Design review of the part built by this model. Coordinates are the model's own, in mm. A direction names the side the tool comes from. Round coordinates to 2 decimals unless told otherwise and drop trailing zeros. Order: outer loops, then holes, each group sorted by start corner. A loop starts at its lowest first (then second) coordinate and runs counter-clockwise, first axis right, second up.
from build123d import *

# Parameters (mm, degrees)
SKETCH1_R           = 2.2
BOSS_EXTRUDE1_DEPTH = 2.38125
BOSS_EXTRUDE3_DEPTH = 2.38125
SKETCH4_R           = 2.15265
CUT_EXTRUDE1_DEPTH  = 2.38125
FILLET2_R           = 2.38125


with BuildPart() as part:
    # Sketch1 → Boss-Extrude1 (new body)
    # profile 1 of 2: a face of its own
    with BuildSketch(Plane(origin=(0, 0, 0), x_dir=(1, 0, 0), z_dir=(0, 1, 0))):
        Polygon((0, -6.985), (0, 0), (-20.15, 0), (-20.15, 20), (-27.65, 20), (-27.65, -6.985), align=None)
        with Locations(Location((-23.9, 4.9, 0), (0, 0, 90))):
            Circle(SKETCH1_R, mode=Mode.SUBTRACT)
        with Locations(Location((-23.9, 15.1, 0), (0, 0, 90))):
            Circle(SKETCH1_R, mode=Mode.SUBTRACT)
    # profile 2 of 2: a face of its own
    with BuildSketch(Plane(origin=(0, 0, 0), x_dir=(1, 0, 0), z_dir=(0, 1, 0))):
        Polygon((20.15, 20), (20.15, 0), (0, 0), (0, -6.985), (27.65, -6.985), (42.38375, -6.985), (42.38375, 20), align=None)
        with Locations(Location((23.9, 4.9, 0), (0, 0, 90))):
            Circle(SKETCH1_R, mode=Mode.SUBTRACT)
        with Locations(Location((23.9, 15.1, 0), (0, 0, 90))):
            Circle(SKETCH1_R, mode=Mode.SUBTRACT)
    extrude(amount=BOSS_EXTRUDE1_DEPTH)

    # Sketch3 → Boss-Extrude3 (add)
    with BuildSketch(Plane(origin=(42.38375, 0, 0), x_dir=(0, 0, -1), z_dir=(1, 0, 0))):
        Polygon((20, 0), (3.015, -37.61875), (-6.985, -37.61875), (-6.985, 2.38125), (20, 2.38125), align=None)
    extrude(amount=BOSS_EXTRUDE3_DEPTH)

    # Sketch4 → Cut-Extrude1 (cut)
    with BuildSketch(Plane(origin=(44.765, 0, 0), x_dir=(0, 0, -1), z_dir=(1, 0, 0))):
        with Locations((-1.397, -13.64595)):
            Circle(SKETCH4_R)
        with Locations((-1.397, -32.69595)):
            Circle(SKETCH4_R)
    extrude(amount=-CUT_EXTRUDE1_DEPTH, mode=Mode.SUBTRACT)

    # Fillet2
    fillet2_edges = [part.edges().sort_by_distance(p)[0] for p in [
        (-27.65, 1.190625, 6.985),
        (-27.65, 1.190625, -20),
        (-20.15, 1.190625, -20),
        (20.15, 1.190625, -20),
        (43.574375, -37.61875, 6.985),
        (43.574375, -37.61875, -3.015),
    ]]
    fillet(fillet2_edges, radius=FILLET2_R)


solid = part.part
1) Clearance check with flat-ended pins moving along their axes: P1, Ø13.5, axis at x = 5, z = -11.5, coming from the -Y side; P2, Ø1.5, axis at x = -18, z = 3.5, coming from the -Y side; P3, Ø0.7, axis at x = 8, y = 1.5, coming from the -Z side; P4, Ø5, axis at y = -32.7, z = 1.4, coming from the -X side. State where each tip first meets the part, or that it passes through.
Results:
P1: passes through
P2: stops at y = 0
P3: stops at z = 0
P4: stops at x = 42.38
2) Take a section at D-D on z = -8.25. Give the boundary of the cut face in (x, y) (3 decimals), plus the area to 3 significant figures.
Results:
outline: (-27.65, 0) - (-20.15, 0) - (-20.15, 2.381) - (-27.65, 2.381) - close; (20.15, 0) - (42.384, 0) - (42.384, -26.024) - (44.765, -26.024) - (44.765, 2.381) - (20.15, 2.381) - close
area: 138 mm2
3) Take a section at A-A on x = 23.9. Give the boundary of the cut face in (y, z) (3 decimals), plus the area to 3 significant figures.
Results:
outline: (0, -20) - (2.381, -20) - (2.381, -17.3) - (0, -17.3) - close; (0, -12.9) - (2.381, -12.9) - (2.381, -7.1) - (0, -7.1) - close; (0, -2.7) - (2.381, -2.7) - (2.381, 6.985) - (0, 6.985) - close
area: 43.3 mm2
4) Take a section at B-B on y = -33.5. Give the boundary of the cut face in (x, z) (3 decimals), plus the area to 3 significant figures.
Results:
outline: (42.384, -4.875) - (44.765, -4.875) - (44.765, -0.6) - (42.384, -0.6) - close; (42.384, 3.394) - (44.765, 3.394) - (44.765, 6.985) - (42.384, 6.985) - close
area: 18.7 mm2
5) The part is to be moulded in two halves that separate along X. For faces 1 (the face through (33, 1, -20)), 2 (the face through (44.765, -13, -4)), 3 (the face through (20.866, 1.207, -19.321)), say which applies: released by +X, released by -X, zero draft, split by the parting line, or undercut.
Results:
face 1: zero draft
face 2: released by +X
face 3: undercut
6) To check wall thickness, follow line 1 along X through (y, z) = (1.7, -15.1) (3 decimals); line 2 along Z through (x, y) = (-23.9, 1.35) (3 decimals); line 3 along Y through (x, z) = (-25, -13). State the ranges of each line that lie inside material, in increasing order.
Results:
line 1: x = -27.65 to -26.1, -21.7 to -20.15, 20.15 to 21.7, 26.1 to 44.765
line 2: z = -20 to -17.3, -12.9 to -7.1, -2.7 to 6.985
line 3: y = 0 to 2.38
7) Take a section at C-C on z = -15.1. Give the boundary of the cut face in (x, y) (3 decimals), plus the area to 3 significant figures.
Results:
outline: (-27.65, 0) - (-26.1, 0) - (-26.1, 2.381) - (-27.65, 2.381) - close; (-21.7, 0) - (-20.15, 0) - (-20.15, 2.381) - (-21.7, 2.381) - close; (20.15, 0) - (21.7, 0) - (21.7, 2.381) - (20.15, 2.381) - close; (26.1, 0) - (42.384, 0) - (42.384, -10.853) - (44.765, -10.853) - (44.765, 2.381) - (26.1, 2.381) - close
area: 81.4 mm2
8) For faces 4 (the face through (20.15, 1, -9)), 5 (the face through (-25.39, 1.17, -3.28)), 6 (the face through (15, 0, 2)), list the 3-axis set-ups (+Z, -Z, +X, -X, +Y, -Y) from which the entire face can be reached by the end or side of a thin tool; tool diameter is ignored.
Results:
face 4: -Z, +Y, -Y
face 5: +Y, -Y
face 6: +Z, -Z, -X, -Y
